from build123d import *

# Parameters (mm, degrees)
HOLE_WIZARD_M41_D = 3.3


with BuildPart() as part:
    # Эскиз2 → Повернуть1 (revolve)
    with BuildSketch(Plane.XY, mode=Mode.PRIVATE) as revolve_1_sk:
        Polygon((1.5, -0.122080905), (3.5, -0.122080905), (3.5, 1.677919095), (3, 1.677919095), (3, 2.277919095), (3.25, 2.277919095), (3.25, 3.477919095), (2.75, 4.077919095), (2.75, 4.877919095), (3, 4.877919095), (3, 5.377919095), (2.5, 5.877919095), (1.5, 5.877919095), align=None)
    revolve(revolve_1_sk.sketch.rotate(Axis((0, 0, 0), (0, 1, 0)), 90), axis=Axis((0, 0, 0), (0, 1, 0)))

    # Отверстие обработанное метчиком M41 (through all)
    with Locations(Plane(origin=(0, -0.122080905, 0), x_dir=(-1, 0, 0), z_dir=(0, -1, 0))):
        with Locations((0, 0)):
            Hole(HOLE_WIZARD_M41_D / 2)


solid = part.part
Can you work these out from the model? Positions are in its coordinate system, mm. A direction names the side the tool comes from. Coordinates: 2 decimals unless noted, no trailing zeros. Loops run counter-clockwise (first coordinate to the right, second up) from the corner with the lowest first, then second, coordinate; pieces in that order, holes last. Notation, with made-up numbers: (30.5, 72) - (60.5, 72) arc R22 ccw to (60.5, 79) - close; hole circle Ø4 at (3.5, 23.5). An arc over 180 degrees is marked (long way). Answer as a JSON object with one key per item and string values. Group by question number.
Item 1: If we section it at C-C (y = 3): List the corners of the cut face in (x, z) for me.
Item 2: If we section it at D-D (y = 4.25): List the corners of the cut face in (x, z) for me.
Item 3: If I drill on L1, parallel to X at y = 2.5, z = 1.5; L2, parallel to X at y = 4.75, z = -0.25; L3, parallel to Z at x = 1.5, y = 1.25, over which ranges is the centre line in solid material (lowest first)? Write a range as from..to.
Item 4: If we section it at B-B (z = 0): List the corners of the cut face in (x, y) for me, plus the area to 4 significant figures.
Item 5: For pin 1 (2 mm diameter, centred on x = -1.5, y = 2, fed in from -Z); pin 2 (3 mm diameter, centred on x = 1.5, y = 3, fed in from -Z); pin 3 (1.5 mm diameter, centred on x = -1.5, y = 5, fed in from -Z), each with a flat end and sliding along its axis, tell me the tip position at first contact or that it passes through.
Item 6: If we section it at A-A (x = 0): List the corners of the cut face in (y, z) for me, plus the area to 4 significant figures.
Item 7: On a 3-axis mill with a long thin cutter (end or side, diameter ignored), from which of +Z, -Z, +X, -X, +Y, -Y can I reach the whole of each face in a straight line? I mean faces 1 (the face through (-1, 1.678, -3)), 2 (the face through (3.105, 0.791, -1.615)), 3 (the face through (-0.9, 5.13, -2.86)). Say none if no direction works.
Item 8: If we mould it in two halves opening along Y, with no side actions, what happens to faces 4 (the face through (2, -0.122, 1)), 5 (the face through (-1.216, 2.92, -1.115)), 6 (the face through (-0.9, 1.98, -2.86))? For each: released by +Y, released by -Y, zero draft, split by the parting line, or undercut.
Returned:
{
 "1": {"outline": "circle Ø6.5 at (0, 0); hole circle Ø3.3 at (0, 0)"},
 "2": {"outline": "circle Ø5.5 at (0, 0); hole circle Ø3.3 at (0, 0)"},
 "3": {"L1": "x = -2.88..-0.69, 0.69..2.88", "L2": "x = -2.74..-1.63, 1.63..2.74", "L3": "z = -3.16..-0.69, 0.69..3.16"},
 "4": {"outline": "(-3.5, -0.12) - (-1.65, -0.12) - (-1.65, 5.88) - (-2.5, 5.88) - (-3, 5.38) - (-3, 4.88) - (-2.75, 4.88) - (-2.75, 4.08) - (-3.25, 3.48) - (-3.25, 2.28) - (-3, 2.28) - (-3, 1.68) - (-3.5, 1.68) - close; (1.65, -0.12) - (3.5, -0.12) - (3.5, 1.68) - (3, 1.68) - (3, 2.28) - (3.25, 2.28) - (3.25, 3.48) - (2.75, 4.08) - (2.75, 4.88) - (3, 4.88) - (3, 5.38) - (2.5, 5.88) - (1.65, 5.88) - close", "area": "17.95 mm²"},
 "5": {"pin 1": "stops at z = -3.46", "pin 2": "stops at z = -3.41", "pin 3": "stops at z = -2.9"},
 "6": {"outline": "(-0.12, -3.5) - (1.68, -3.5) - (1.68, -3) - (2.28, -3) - (2.28, -3.25) - (3.48, -3.25) - (4.08, -2.75) - (4.88, -2.75) - (4.88, -3) - (5.38, -3) - (5.88, -2.5) - (5.88, -1.65) - (-0.12, -1.65) - close; (-0.12, 1.65) - (5.88, 1.65) - (5.88, 2.5) - (5.38, 3) - (4.88, 3) - (4.88, 2.75) - (4.08, 2.75) - (3.48, 3.25) - (2.28, 3.25) - (2.28, 3) - (1.68, 3) - (1.68, 3.5) - (-0.12, 3.5) - close", "area": "17.95 mm²"},
 "7": {"face 1": "none", "face 2": "+Y, -Y", "face 3": "+Y"},
 "8": {"face 4": "released by -Y", "face 5": "zero draft", "face 6": "undercut"}
}
